Here's how the part is built. I have some questions about the finished solid (model axes, mm). A direction names the side the tool comes from. Give positions to 0.01 mm unless a question says otherwise; leave off trailing zeros. Order: outer loops, then holes, each group sorted by start corner. A loop starts at its lowest first (then second) coordinate and runs counter-clockwise, first axis right, second up. Notation, with made-up numbers: M -33,75.25 L 14,75.25 A14 ccw 14,82.25 Z; hole C 18,-17.75 d10. An arc over 180 degrees is marked long. Use one line per item in the form item = value.
from build123d import *

# Parameters (mm, degrees)
SKETCH1_R           = 20
BOSS_EXTRUDE1_DEPTH = 40
SHELL1_T            = -10
BOSS_EXTRUDE2_START = 10
SKETCH1_3_R         = 20
BOSS_EXTRUDE2_DEPTH = 10
SKETCH2_R           = 20
BOSS_EXTRUDE3_DEPTH = 10


with BuildPart() as part:
    # Sketch1 → Boss-Extrude1 (new body)
    # profile 1 of 2: a face of its own
    with BuildSketch(Plane.XY):
        with BuildLine():
            Line((0, 60), (-300, 60))
            ThreePointArc((-300, 60), (-330, 30), (-300, 0))
            Line((-300, 0), (0, 0))
            Line((0, 0), (0, 60))
        make_face()
        with Locations((-300, 30)):
            Circle(SKETCH1_R, mode=Mode.SUBTRACT)
    # profile 2 of 2: a face of its own
    with BuildSketch(Plane.XY):
        with Locations((-300, 30)):
            Circle(SKETCH1_R)
    extrude(amount=-BOSS_EXTRUDE1_DEPTH)

    # Shell1
    shell1_openings = [part.faces().sort_by_distance(p)[0] for p in [
        (0, 30, -20),
    ]]
    offset(amount=SHELL1_T, openings=shell1_openings, kind=Kind.INTERSECTION)

    # Sketch1_3 → Boss-Extrude2 (add)
    with BuildSketch(Plane.XY.offset(BOSS_EXTRUDE2_START)):
        with Locations((-300, 30)):
            Circle(SKETCH1_3_R)
    extrude(amount=-BOSS_EXTRUDE2_DEPTH)

    # Sketch2 → Boss-Extrude3 (add)
    with BuildSketch(Plane(origin=(0, 0, -40), x_dir=(-1, 0, 0), z_dir=(0, 0, -1))):
        with Locations(Location((300, 30, 0), (0, 0, 180))):
            Circle(SKETCH2_R)
    extrude(amount=BOSS_EXTRUDE3_DEPTH)


solid = part.part
Q1. I want a section at D-D on y = 18. Write out the boundary of the cut face in (x, z), then the cut area to 3 significant figures.
Found:
outline = M -327.5,-40 L -316,-40 L -316,-50 L -284,-50 L -284,-40 L 0,-40 L 0,-30 L -316,-30 L -316,-10 L 0,-10 L 0,0 L -284,0 L -284,10 L -316,10 L -316,0 L -327.5,0 Z
area = 7,420 mm²
Q2. Thinking about a two-plate mould opening in Z: for faces 1 (the face through (-300, 30, -50)), 2 (the face through (-329.993, 30.66, -19.72)), 3 (the face through (-162, 30, -30)), which applies, +Z half, -Z half, draft (parallel to the pull), parting line (faces both ways), or undercut?
Found:
face_1 = -Z half
face_2 = draft
face_3 = undercut
Q3. I'm going to push flat-ended pins straight in: pin 1 Ø3 at (x, z) = (-255.5, -10) entering from -Y; pin 2 Ø20 at (x, y) = (-132.5, 30.5) entering from -Z; pin 3 Ø2 at (y, z) = (41.5, -29.5) entering from -X; pin 4 Ø4 at (y, z) = (54, -10.5) entering from -X. Where does each tip first touch, or does it pass through?
Found:
pin_1 = 0
pin_2 = -40
pin_3 = -328.1
pin_4 = -320.4
Q4. I want a section at A-A on y = 30. Write out the boundary of the cut face in (x, z).
Found:
outline = M -330,-40 L -320,-40 L -320,-50 L -280,-50 L -280,-40 L 0,-40 L 0,-30 L -320,-30 L -320,-10 L 0,-10 L 0,0 L -280,0 L -280,10 L -320,10 L -320,0 L -330,0 Z
Q5. I want a section at B-B on x = -149. Write out the boundary of the cut face in (y, z).
Found:
outline = M 0,-40 L 60,-40 L 60,0 L 0,0 Z; hole M 10,-30 L 50,-30 L 50,-10 L 10,-10 Z
Q6. I want a section at C-C on z = -21.5. Write out the boundary of the cut face in (x, y), then the cut area to 3 significant figures.
Found:
outline = M -300,0 L 0,0 L 0,10 L -300,10 A20 cw -300,50 L 0,50 L 0,60 L -300,60 A30 ccw Z
area = 6,790 mm²
Q7. On a 3-axis mill with a long thin cutter (end or side, diameter ignored), from which of +Z, -Z, +X, -X, +Y, -Y can I reach the whole of each face in a straight line? I mean faces 4 (the face through (-300, 30, 10)), 5 (the face through (-281.525, 22.34, 5.07)), 6 (the face through (-281.525, 37.66, -44.93)), 7 (the face through (-148, 50, -20)), 8 (the face through (-148, 60, -20)). Say none if no direction works.
Found:
face_4 = +Z, +X, -X, +Y, -Y
face_5 = +Z
face_6 = -Z
face_7 = +X
face_8 = +Z, -Z, +X, -X, +Y
Q8. I need wall thicknesses on L1, parallel to Y at x = -29, z = -14.5; L2, parallel to Z at x = -285, y = 31; L3, parallel to Z at x = -33.5, y = 46.5. Which ranges of each line are inside material? Lowest first, please.
Found:
L1 = 0 to 10, 50 to 60
L2 = -50 to -30, -10 to 10
L3 = -40 to -30, -10 to 0
